from build123d import *

# Parameters (mm, degrees)
EXTRUDE_1_DEPTH             = 50
SKETCH_2_W                  = 20.000664015
SKETCH_2_H                  = 5
EXTRUDE_2_DEPTH             = 240
EXTRUDE_3_DEPTH             = 50
EXTRUDE_3_DEPTH_BACK        = 100
SKETCH_3_W                  = 25
SKETCH_3_H                  = 5
RIB_2_REACH                 = 314.17
SKETCH_4_WALL_W             = 700.669994888
SKETCH_4_WALL_H             = 10
RIB_3_REACH                 = 314.17
SKETCH_5_WALL_W             = 700.669994888
SKETCH_5_WALL_H             = 10
CUT_EXTRUDE_START           = -190
SKETCH_6_W                  = 20
SKETCH_6_H                  = 65
CUT_EXTRUDE_1_DEPTH         = 190
SKETCH_7_W                  = 100
SKETCH_7_H                  = 20
CUT_EXTRUDE_2_DEPTH         = 5
EXTRUDE_5_DEPTH             = 5
MIRROR_2_COPY_1_DEPTH       = 5
EXTRUDE_6_REACH             = 244.126
SKETCH_10_W                 = 5
SKETCH_10_H                 = 5
EXTRUDE_6_DIRECTION_2_REACH = 244.126
FILLET_1_R                  = 5
FILLET_2_R                  = 5
FILLET_3_R                  = 5
FILLET_4_R                  = 5
FILLET_5_R                  = 10
FILLET_6_R                  = 5


with BuildPart() as part:
    # 草图1 → 凸台-拉伸1 (new body)
    with BuildSketch(Plane.XY):
        Polygon((0, 0), (30, 0), (30, 180), (50, 180), (50, 160), (190, 160), (190, 180), (210, 180), (210, 0), (240, 0), (240, 5), (215, 5), (215, 185), (185, 185), (185, 165), (55, 165), (55, 185), (25, 185), (25, 5), (0, 5), align=None)
    extrude(amount=EXTRUDE_1_DEPTH)

    # 草图2 → 凸台-拉伸2 (add)
    with BuildSketch(Plane.ZY):
        with Locations((25.000332008, 2.5)):
            Rectangle(SKETCH_2_W, SKETCH_2_H)
    extrude(amount=-EXTRUDE_2_DEPTH)

    # 草图3 → 凸台-拉伸3 (add, two sides: drawn at the far end of the back side and taken through both)
    with BuildSketch(Plane(origin=(0, 0, 0), x_dir=(-1, 0, 0), z_dir=(0, 0, -1)).offset(-EXTRUDE_3_DEPTH_BACK)):
        with Locations((-227.5, 2.5)):
            Rectangle(SKETCH_3_W, SKETCH_3_H)
        with Locations((-12.5, 2.5)):
            Rectangle(SKETCH_3_W, SKETCH_3_H)
    extrude(amount=EXTRUDE_3_DEPTH + EXTRUDE_3_DEPTH_BACK)

    # 草图4 wall → 筋2 (add, up to next)
    with BuildSketch(Plane(origin=(227.5, 40, 25), x_dir=(-0.336336396998, 0.941741911595, 0), z_dir=(0.941741911595, 0.336336396998, 0)), mode=Mode.PRIVATE) as rib_2_sk1:
        Rectangle(SKETCH_4_WALL_W, SKETCH_4_WALL_H)
    rib_2_tool1 = extrude(rib_2_sk1.sketch, amount=-RIB_2_REACH, mode=Mode.PRIVATE) - part.part
    add(rib_2_tool1.solids().sort_by_distance((227.5, 40, 25))[0])

    # 草图5 wall → 筋3 (add, up to next)
    with BuildSketch(Plane(origin=(12.5, 40, 25), x_dir=(-0.336336396998, -0.941741911595, 0), z_dir=(-0.941741911595, 0.336336396998, 0)), mode=Mode.PRIVATE) as rib_3_sk1:
        Rectangle(SKETCH_5_WALL_W, SKETCH_5_WALL_H)
    rib_3_tool1 = extrude(rib_3_sk1.sketch, amount=-RIB_3_REACH, mode=Mode.PRIVATE) - part.part
    add(rib_3_tool1.solids().sort_by_distance((12.5, 40, 25))[0])

    # 草图6 → 切除-拉伸1 (cut)
    with BuildSketch(Plane(origin=(215, 0, 0), x_dir=(0, 0, -1), z_dir=(1, 0, 0)).offset(CUT_EXTRUDE_START)):
        with Locations((-25, 117.5)):
            Rectangle(SKETCH_6_W, SKETCH_6_H)
    extrude(amount=CUT_EXTRUDE_1_DEPTH, mode=Mode.SUBTRACT)

    # 草图7 → 切除-拉伸2 (cut)
    with BuildSketch(Plane(origin=(0, 165, 0), x_dir=(1, 0, 0), z_dir=(0, 1, 0))):
        with Locations((120, -25)):
            Rectangle(SKETCH_7_W, SKETCH_7_H)
    extrude(amount=-CUT_EXTRUDE_2_DEPTH, mode=Mode.SUBTRACT)

    # 草图9 → 凸台-拉伸5 (add)
    with BuildSketch(Plane(origin=(0, 0, 0), x_dir=(-1, 0, 0), z_dir=(0, 0, -1))):
        Polygon((-190, 160), (-210, 137.300480815), (-210, 148.645505565), (-190, 171.34502475), align=None)
    extrude_5 = extrude(amount=-EXTRUDE_5_DEPTH)

    # 镜向1: 凸台-拉伸5 across plane
    add(extrude_5.mirror(Plane(origin=(0, 0, 25), x_dir=(1, 0, 0), z_dir=(0, 0, -1))))

    # 镜向2: 凸台-拉伸5 across plane
    add(extrude_5.mirror(Plane(origin=(120, 0, 0), x_dir=(0, 0, 1), z_dir=(1, 0, 0))))

    # 镜向2 copy 1 sketch → 镜向2 copy 1 (add)
    with BuildSketch(Plane(origin=(240, 0, 50), x_dir=(1, 0, 0), z_dir=(0, 0, 1))):
        Polygon((-190, 160), (-210, 137.300480815), (-210, 148.645505565), (-190, 171.34502475), align=None)
    extrude(amount=-MIRROR_2_COPY_1_DEPTH)

    # 凸台-拉伸6: up to this face of the body (flat: up to its plane)
    extrude_6_end = Plane(part.part.faces().sort_by_distance((170, 162.5, 25))[0])
    # 草图10 → 凸台-拉伸6 (add, up to the picked face)
    with BuildSketch(Plane(origin=(120, 0, 0), x_dir=(0, 0, -1), z_dir=(1, 0, 0)), mode=Mode.PRIVATE) as extrude_6_sk1:
        with Locations((-47.5, 157.5)):
            Rectangle(SKETCH_10_W, SKETCH_10_H)
    extrude_6_tool1 = split(extrude(extrude_6_sk1.sketch, amount=EXTRUDE_6_REACH, mode=Mode.PRIVATE), bisect_by=extrude_6_end, keep=Keep.BOTH, mode=Mode.PRIVATE)
    extrude_6 = extrude_6_tool1.solids().sort_by(Axis((120, 157.5, 47.5), (1, 0, 0)))[0]
    add(extrude_6)

    # 凸台-拉伸6 direction 2: up to this face of the body (flat: up to its plane)
    extrude_6_direction_2_end = Plane(part.part.faces().sort_by_distance((70, 162.5, 25))[0])
    # 草图10 → 凸台-拉伸6 direction 2 (add, up to the picked face)
    with BuildSketch(Plane(origin=(120, 0, 0), x_dir=(0, 0, -1), z_dir=(1, 0, 0)), mode=Mode.PRIVATE) as extrude_6_direction_2_sk1:
        with Locations((-47.5, 157.5)):
            Rectangle(SKETCH_10_W, SKETCH_10_H)
    extrude_6_direction_2_tool1 = split(extrude(extrude_6_direction_2_sk1.sketch, amount=-EXTRUDE_6_DIRECTION_2_REACH, mode=Mode.PRIVATE), bisect_by=extrude_6_direction_2_end, keep=Keep.BOTH, mode=Mode.PRIVATE)
    extrude_6_direction_2 = extrude_6_direction_2_tool1.solids().sort_by(Axis((120, 157.5, 47.5), (-1, 0, 0)))[0]
    add(extrude_6_direction_2)

    # 镜向3: 凸台-拉伸6, 凸台-拉伸6 direction 2 across plane
    add(extrude_6.mirror(Plane(origin=(0, 0, 25), x_dir=(1, 0, 0), z_dir=(0, 0, -1))))
    add(extrude_6_direction_2.mirror(Plane(origin=(0, 0, 25), x_dir=(1, 0, 0), z_dir=(0, 0, -1))))

    # 圆角1
    fillet_1_edges = [part.edges().sort_by_distance(p)[0] for p in [
        (70, 160, 47.5),
    ]]
    fillet(fillet_1_edges, radius=FILLET_1_R - 0.0001)  # a hair under: the kernel refuses the full size

    # 圆角2
    fillet_2_edges = [part.edges().sort_by_distance(p)[0] for p in [
        (170, 160, 47.5),
    ]]
    fillet(fillet_2_edges, radius=FILLET_2_R - 0.0001)  # a hair under: the kernel refuses the full size

    # 圆角3
    fillet_3_edges = [part.edges().sort_by_distance(p)[0] for p in [
        (170, 160, 2.5),
    ]]
    fillet(fillet_3_edges, radius=FILLET_3_R - 0.0001)  # a hair under: the kernel refuses the full size

    # 圆角4
    fillet_4_edges = [part.edges().sort_by_distance(p)[0] for p in [
        (70, 160, 2.5),
    ]]
    fillet(fillet_4_edges, radius=FILLET_4_R - 0.0001)  # a hair under: the kernel refuses the full size

    # 圆角5
    fillet_5_edges = [part.edges().sort_by_distance(p)[0] for p in [
        (215, 2.5, 100),
        (215, 2.5, -50),
        (25, 2.5, 100),
        (25, 2.5, -50),
        (25, 185, 25),
        (55, 185, 25),
        (185, 185, 25),
        (215, 185, 25),
    ]]
    fillet(fillet_5_edges, radius=FILLET_5_R)

    # 圆角6
    fillet_6_edges = [part.edges().sort_by_distance(p)[0] for p in [
        (240, 2.5, 100),
        (240, 2.5, -50),
        (0, 2.5, 100),
        (0, 2.5, -50),
    ]]
    fillet(fillet_6_edges, radius=FILLET_6_R)


solid = part.part
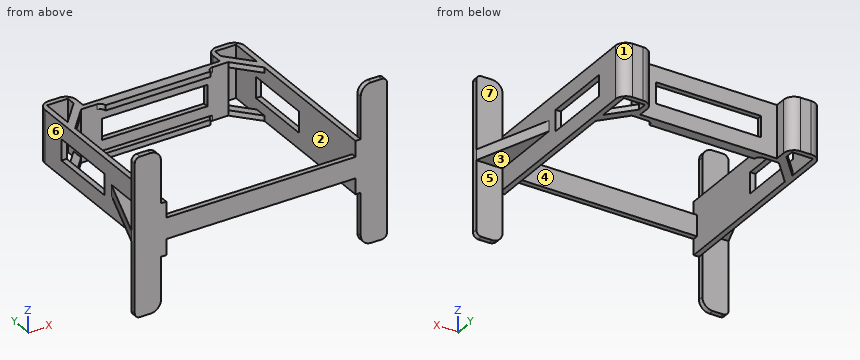
Source: CAD feature listing. Evaluate the final solid. Frame: model axes, mm. Face numbers are marked on the shaded views. A direction names the side the tool comes from. Round coordinates to 2 decimals unless told otherwise and drop trailing zeros. Loops run counter-clockwise (first coordinate to the right, second up) from the corner with the lowest first, then second, coordinate; pieces in that order, holes last. Notation, with made-up numbers: (61, -37) -> (91, -37) arc R35 cw to (91, -4) -> close; hole circle Ø2 at (-36.5, 8). An arc over 180 degrees is marked (long way). Answer as a JSON object with one key per item and string values. Group by question number.
Q1. Mould query, pull axis X, two halves, no side actions, for the marked faces 1, 2 and 3. Classes: pulls with the +X half, pulls with the -X half, needs draft (parallel to the pull), parting line crosses it, or undercut.
Q2. Section query B-B (y = 43.5). Output: boundary loops of the cut face in (x, z), plus the area to 3 significant figures.
Q3. Section query A-A (x = 180). Output: boundary loops of the cut face in (y, z), plus the area to 3 significant figures.
Q4. Section query D-D (z = 80.5). Output: boundary loops of the cut face in (x, y), plus the area to 3 significant figures.
Q5. Section query C-C (y = 117.5). Output: boundary loops of the cut face in (x, z), plus the area to 3 significant figures.
Q6. Contact query for flat-ended pins moving along their axis: P1, Ø16, axis at x = 203, z = 25, coming from the -Y side; P2, Ø1.5, axis at x = 149, z = 3.5, coming from the -Y side; P3, Ø20, axis at x = 8, y = 50, coming from the -Z side; P4, Ø5.5, axis at y = 162, z = 26.5, coming from the -X side. Output: stop coordinate, or through.
Q7. Ray query, line 1 (Y direction, x = 180.5, z = 34); line 2 (X direction, y = 62.5, z = 43); line 3 (Y direction, x = 216, z = 82.5). Return the intervals inside material, ascending. Write a range as from..to.
Q8. Access query for the marked faces 4, 5, 6 and 7. Directions: +Z, -Z, +X, -X, +Y, -Y. A direction counts if a zero-diameter tool reaches every point of the face in a straight line with its end or side. Return the directions, or none.
Completed:
{
 "1": {"face 1": "pulls with the +X half", "face 2": "undercut", "face 3": "needs draft"},
 "2": {"outline": "(13.75, 20) -> (25, 20) -> (25, 0) -> (30, 0) -> (30, 50) -> (25, 50) -> (25, 30) -> (13.75, 30) -> close; (210, 0) -> (215, 0) -> (215, 20) -> (226.25, 20) -> (226.25, 30) -> (215, 30) -> (215, 50) -> (210, 50) -> close", "area": "725 mm²"},
 "3": {"outline": "(0, 15) -> (5, 15) -> (5, 35) -> (0, 35) -> close; (160, 0) -> (165, 0) -> (165, 50) -> (160, 50) -> close", "area": "350 mm²"},
 "4": {"outline": "(0, 0) -> (25, 0) -> (25, 5) -> (0, 5) -> close; (215, 0) -> (240, 0) -> (240, 5) -> (215, 5) -> close", "area": "250 mm²"},
 "5": {"outline": "(25, 0) -> (30, 0) -> (30, 15) -> (25, 15) -> close; (25, 35) -> (30, 35) -> (30, 50) -> (25, 50) -> close; (210, 0) -> (215, 0) -> (215, 15) -> (210, 15) -> close; (210, 35) -> (215, 35) -> (215, 50) -> (210, 50) -> close", "area": "300 mm²"},
 "6": {"P1": "y = 0", "P2": "y = 155", "P3": "z = 20", "P4": "x = 25"},
 "7": {"line 1": "0..5, 160..165", "line 2": "25..30, 210..215", "line 3": "0..5"},
 "8": {"face 4": "+Z, -Z", "face 5": "-Z, +X, +Y", "face 6": "-X, +Y", "face 7": "+Z, +X, +Y"}
}
